from build123d import *

# Parameters (mm, degrees)
F1_DEPTH  = 100
F3_DEPTH  = 330.001
F4_W      = 12.2
F4_H      = 28
F5_DEPTH  = 25
F6_DEPTH  = 6
F7_DEPTH  = 6
F9_DEPTH  = 4
F8_R      = 1.25
F10_DEPTH = 25


with BuildPart() as f1:
    # F0 (on Top) → F1 (new body)
    with BuildSketch(Plane.XY):
        with BuildLine():
            ThreePointArc((0, 12.5), (3.6611652352, 3.6611652352), (12.5, 0))
            Line((12.5, 0), (137.5, 0))
            ThreePointArc((137.5, 0), (146.3388347648, 3.6611652352), (150, 12.5))
            Line((150, 12.5), (150, 317.5))
            ThreePointArc((150, 317.5), (146.3388347648, 326.3388347648), (137.5, 330))
            Line((137.5, 330), (12.5, 330))
            ThreePointArc((12.5, 330), (3.6611652352, 326.3388347648), (0, 317.5))
            Line((0, 317.5), (0, 12.5))
        make_face()
        with BuildLine():
            ThreePointArc((12.5, 4), (6.4895923599, 6.4895923599), (4, 12.5))
            Line((4, 12.5), (4, 317.5))
            ThreePointArc((4, 317.5), (6.4895923599, 323.5104076401), (12.5, 326))
            Line((12.5, 326), (137.5, 326))
            ThreePointArc((137.5, 326), (143.5104076401, 323.5104076401), (146, 317.5))
            Line((146, 317.5), (146, 12.5))
            ThreePointArc((146, 12.5), (143.5104076401, 6.4895923599), (137.5, 4))
            Line((137.5, 4), (12.5, 4))
        make_face(mode=Mode.SUBTRACT)
    extrude(amount=F1_DEPTH)

    # F2 (on face) → F3 (cut, through all)
    with BuildSketch(Plane.XZ):
        with BuildLine():
            Line((109.958435546, 80), (40, 80))
            ThreePointArc((40, 80), (22.5008510571, 62.3274129951), (40.3451572234, 45.0034041456))
            Line((40.3451572234, 45.0034041456), (109.9991571426, 45.0000493805))
            ThreePointArc((109.9991571426, 45.0000493805), (127.4999999949, 62.4996279315), (110, 80.0000493602))
            ThreePointArc((110, 80.0000493602), (109.9792177583, 80.0000370201), (109.958435546, 80))
        make_face()
    extrude(amount=-F3_DEPTH, mode=Mode.SUBTRACT)

    # F4 (on face) → F5 (cut)
    with BuildSketch(Plane.YZ.offset(150)):
        with Locations((291.4, 36)):
            Rectangle(F4_W, F4_H)
    extrude(amount=-F5_DEPTH, mode=Mode.SUBTRACT)

    # F6 (add): a face of the model
    f6_faces = [f1.faces().sort_by_distance(p)[0] for p in [
        (148, 291.4, 22),
    ]]
    extrude(f6_faces, amount=F6_DEPTH)

    # F7 (cut): a face of the model
    f7_faces = [f1.faces().sort_by_distance(p)[0] for p in [
        (148, 291.4, 50),
    ]]
    extrude(f7_faces, amount=-F7_DEPTH, mode=Mode.SUBTRACT)

    # F8 (on face) → F9 (cut, through all)
    with BuildSketch(Plane(origin=(0, 0, 0), x_dir=(0, -1, 0), z_dir=(-1, 0, 0))):
        with BuildLine():
            Line((-290.5, 34.75), (-297.5, 34.75))
            ThreePointArc((-297.5, 34.75), (-302.25, 30), (-297.5, 25.25))
            Line((-297.5, 25.25), (-290.5, 25.25))
            Line((-290.5, 25.25), (-290.5, 34.75))
        make_face()
    extrude(amount=-F9_DEPTH, mode=Mode.SUBTRACT)

    # F8 (on face) → F10 (cut)
    with BuildSketch(Plane(origin=(0, 0, 0), x_dir=(0, -1, 0), z_dir=(-1, 0, 0))):
        with BuildLine():
            Line((-290.5, 34.75), (-297.5, 34.75))
            ThreePointArc((-297.5, 34.75), (-302.25, 30), (-297.5, 25.25))
            Line((-297.5, 25.25), (-290.5, 25.25))
            Line((-290.5, 25.25), (-290.5, 34.75))
        make_face()
        with Locations((-304.25, 30)):
            Circle(F8_R)
        with Locations((-288.35, 30)):
            Circle(F8_R)
    extrude(amount=-F10_DEPTH, mode=Mode.SUBTRACT)


solid = f1.part
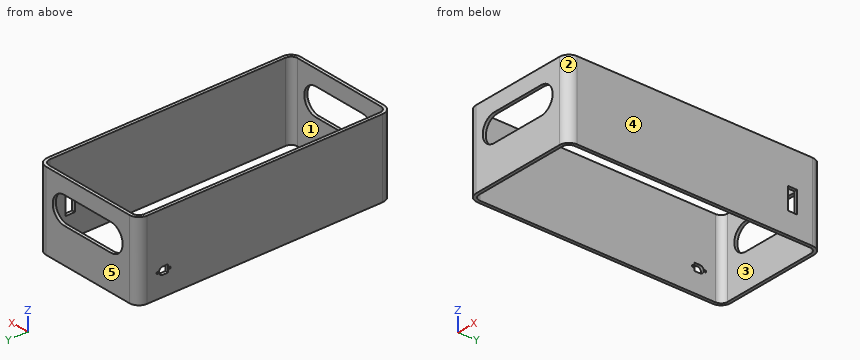
The model under review builds one solid part; all positions refer to its coordinate system, in mm. Face numbers are marked on the shaded views. A direction names the side the tool comes from. Coordinates: 2 decimals unless noted, no trailing zeros. Loops run counter-clockwise (first coordinate to the right, second up) from the corner with the lowest first, then second, coordinate; pieces in that order, holes last. Notation, with made-up numbers: (-17, 24.5) -> (-8, 24.5) arc R27 ccw to (-8, 63.5) -> close; hole circle Ø6 at (-14, 42). An arc over 180 degrees is marked (long way). Use a Markdown table: item, result. Add a question column.
1. Add section C-C on x = 85.5. Write out the cut boundary in (y, z), plus the area to 3 significant figures.
2. Add section B-B on y = 152. Write out the cut boundary in (x, z), plus the area to 3 significant figures.
3. Add section D-D on z = 9.5. Write out the cut boundary in (x, y).
4. To check wall thickness, follow line 1 (X direction, y = 114, z = 54.5); line 2 (Z direction, x = 2, y = 304); line 3 (Y direction, x = 63.5, z = 91). State the ranges of each line that lie inside material, in increasing order.
5. Add section A-A on z = 62.5. Write out the cut boundary in (x, y), plus the area to 3 significant figures.
6. Clearance check with flat-ended pins moving along their axes: pin 1 Ø3 at (x, z) = (148.5, 47) entering from -Y; pin 2 Ø4.5 at (x, z) = (147.5, 47) entering from +Y. State where each tip first meets the part, or that it passes through.
7. Machinability: for the marked faces 1 and 2, which of the approach directions +Z, -Z, +X, -X, +Y, -Y give a long, thin tool a straight path to every point of the face, cutting with its end or side? Answer none if there is none.
8. Draft analysis for pull direction X (two halves, no side actions). For the marked faces 3, 4 and 5, state which applies: pulls with the +X half, pulls with the -X half, needs draft (parallel to the pull), parting line crosses it, or undercut.
Returned:
| question | item | result |
|---|---|---|
| 1 | outline | (0, 0) -> (4, 0) -> (4, 45) -> (0, 45) -> close; (0, 80) -> (4, 80) -> (4, 100) -> (0, 100) -> close; (326, 0) -> (330, 0) -> (330, 45) -> (326, 45) -> close; (326, 80) -> (330, 80) -> (330, 100) -> (326, 100) -> close |
| 1 | area | 520 mm² |
| 2 | outline | (0, 0) -> (4, 0) -> (4, 100) -> (0, 100) -> close; (146, 0) -> (150, 0) -> (150, 100) -> (146, 100) -> close |
| 2 | area | 800 mm² |
| 3 | outline | (0, 12.5) arc R12.5 ccw to (12.5, 0) -> (137.5, 0) arc R12.5 ccw to (150, 12.5) -> (150, 317.5) arc R12.5 ccw to (137.5, 330) -> (12.5, 330) arc R12.5 ccw to (0, 317.5) -> close; hole (4, 12.5) arc R8.5 ccw to (12.5, 4) -> (137.5, 4) arc R8.5 ccw to (146, 12.5) -> (146, 317.5) arc R8.5 ccw to (137.5, 326) -> (12.5, 326) arc R8.5 ccw to (4, 317.5) -> close |
| 4 | line 1 | x = 0 to 4, 146 to 150 |
| 4 | line 2 | z = 0 to 28.78, 31.22 to 100 |
| 4 | line 3 | y = 0 to 4, 326 to 330 |
| 5 | outline | (0, 12.5) arc R12.5 ccw to (12.5, 0) -> (22.5, 0) -> (22.5, 4) -> (12.5, 4) arc R8.5 cw to (4, 12.5) -> (4, 317.5) arc R8.5 cw to (12.5, 326) -> (22.5, 326) -> (22.5, 330) -> (12.5, 330) arc R12.5 ccw to (0, 317.5) -> close; (127.5, 0) -> (137.5, 0) arc R12.5 ccw to (150, 12.5) -> (150, 317.5) arc R12.5 ccw to (137.5, 330) -> (127.5, 330) -> (127.5, 326) -> (137.5, 326) arc R8.5 cw to (146, 317.5) -> (146, 12.5) arc R8.5 cw to (137.5, 4) -> (127.5, 4) -> close |
| 5 | area | 2,860 mm² |
| 6 | pin 1 | stops at y = 4.38 |
| 6 | pin 2 | stops at y = 327.31 |
| 7 | face 1 | +Z, -Z |
| 7 | face 2 | +Z, -Z, +X, -Y |
| 8 | face 3 | undercut |
| 8 | face 4 | pulls with the +X half |
| 8 | face 5 | needs draft |
